from build123d import *

# Parameters (mm, degrees)
SKETCH1_W           = 1311.148
SKETCH1_H           = 701.548
BOSS_EXTRUDE1_DEPTH = 542.544
CUT_EXTRUDE1_START  = 542.544
SKETCH1_4_W         = 1234.948
SKETCH1_4_H         = 625.348
CUT_EXTRUDE1_DEPTH  = 448.818


with BuildPart() as part:
    # Sketch1 → Boss-Extrude1 (new body)
    with BuildSketch(Plane(origin=(0, 0, 0), x_dir=(1, 0, 0), z_dir=(0, 1, 0))):
        Rectangle(SKETCH1_W, SKETCH1_H)
    extrude(amount=BOSS_EXTRUDE1_DEPTH)

    # Sketch1<4> → Cut-Extrude1 (cut)
    with BuildSketch(Plane(origin=(0, 0, 0), x_dir=(1, 0, 0), z_dir=(0, 1, 0)).offset(CUT_EXTRUDE1_START)):
        Rectangle(SKETCH1_4_W, SKETCH1_4_H)
    extrude(amount=-CUT_EXTRUDE1_DEPTH, mode=Mode.SUBTRACT)


solid = part.part
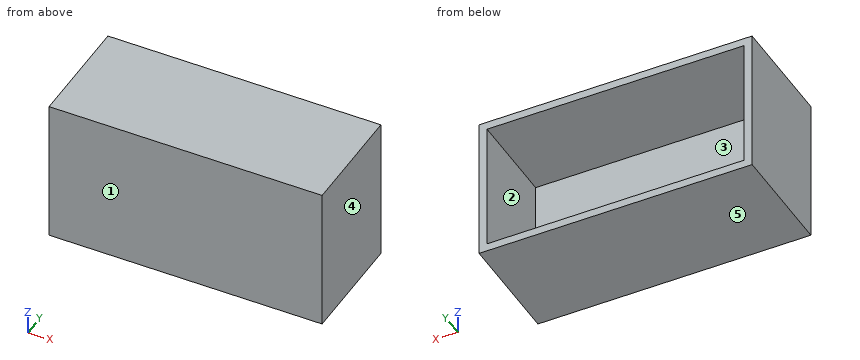
Could you check a few things on this model? Use its own coordinates, in mm. Face numbers are marked on the shaded views. A direction names the side the tool comes from. Give positions to 0.01 mm unless a question says otherwise; leave off trailing zeros. Order: outer loops, then holes, each group sorted by start corner. A loop starts at its lowest first (then second) coordinate and runs counter-clockwise, first axis right, second up. Notation, with made-up numbers: (58.5, 49.5) -> (93.5, 49.5) arc R16 ccw to (93.5, 80.5) -> close; hole circle Ø8 at (82, 14.5). An arc over 180 degrees is marked (long way). Return JSON: item names as keys, results as strings.
1. On a 3-axis mill with a long thin cutter (end or side, diameter ignored), from which of +Z, -Z, +X, -X, +Y, -Y can I reach the whole of each face in a straight line? I mean the marked faces 1 and 2. Say none if no direction works.
Answer list:
{"face 1": "+Z, -Z, +X, -X, -Y", "face 2": "+Y"}
2. Thinking about a two-plate mould opening in Z: for the marked faces 3, 4 and 5, which applies, pulls with the +Z half, pulls with the -Z half, needs draft (parallel to the pull), parting line crosses it, or undercut?
Answer list:
{"face 3": "undercut", "face 4": "needs draft", "face 5": "pulls with the -Z half"}
3. I need wall thicknesses on line 1 (X direction, y = 342.5, z = -183.5); line 2 (Z direction, x = -511.5, y = 421); line 3 (Y direction, x = -49.5, z = -131.5). Which ranges of each line are inside material? Lowest first, please. Write a range as from..to.
Answer list:
{"line 1": "x = -655.57..-617.47, 617.47..655.57", "line 2": "z = -350.77..-312.67, 312.67..350.77", "line 3": "y = 0..93.73"}
4. Imagine slicing it at C-C on x = 379. List the corners of the cut face in (y, z) for me, then the cut area to 4 significant figures.
Answer list:
{"outline": "(0, -350.77) -> (542.54, -350.77) -> (542.54, -312.67) -> (93.73, -312.67) -> (93.73, 312.67) -> (542.54, 312.67) -> (542.54, 350.77) -> (0, 350.77) -> close", "area": "100,000 mm2"}
5. Imagine slicing it at A-A on y = 420. List the corners of the cut face in (x, z) for me.
Answer list:
{"outline": "(-655.57, -350.77) -> (655.57, -350.77) -> (655.57, 350.77) -> (-655.57, 350.77) -> close; hole (-617.47, -312.67) -> (617.47, -312.67) -> (617.47, 312.67) -> (-617.47, 312.67) -> close"}
6. Imagine slicing it at B-B on z = 168. List the corners of the cut face in (x, y) for me.
Answer list:
{"outline": "(-655.57, 0) -> (655.57, 0) -> (655.57, 542.54) -> (617.47, 542.54) -> (617.47, 93.73) -> (-617.47, 93.73) -> (-617.47, 542.54) -> (-655.57, 542.54) -> close"}
7. For pin 1 Ø6 at (x, z) = (83, 228.5) entering from +Y, with a flat end and sliding along its axis, tell me the tip position at first contact or that it passes through.
Answer list:
{"pin 1": "stops at y = 93.73"}
